Could you check a few things on this model? Use its own coordinates, in mm. A direction names the side the tool comes from. Give positions to 0.01 mm unless a question says otherwise; leave off trailing zeros. Write each loop counter-clockwise with the first axis right and the second up, starting at its lowest first coordinate (ties: lowest second). Pieces come first, ordered by that corner, then holes. Notation, with made-up numbers: (52.5, 47.5) - (77.5, 47.5) arc R17 cw to (77.5, 57.5) - close; hole circle Ø10 at (-30, -12.75). An arc over 180 degrees is marked (long way). Use one line per item in the form item = value.
```python
from build123d import *

# Parameters (mm, degrees)
BOSS_EXTRUDE1_DEPTH = 12.6
CUT_EXTRUDE1_DEPTH  = 7
CUT_EXTRUDE2_DEPTH  = 3
SKETCH5_R           = 1
BOSS_EXTRUDE2_DEPTH = 5.9
SKETCH6_R           = 1.25
BOSS_EXTRUDE3_DEPTH = 6.2
SKETCH7_R           = 0.85
CUT_EXTRUDE3_DEPTH  = 4.5
SKETCH8_W           = 3.3
SKETCH8_H           = 2.25
CUT_EXTRUDE4_DEPTH  = 18.024687956
CUT_EXTRUDE5_DEPTH  = 15.941218156
FILLET1_R           = 0.5
FILLET2_R           = 0.25
FILLET3_R           = 0.15
FILLET4_R           = 0.25


with BuildPart() as part:
    # Sketch1 → Boss-Extrude1 (new body)
    with BuildSketch(Plane(origin=(0, 0, 0), x_dir=(0, 0, -1), z_dir=(1, 0, 0))):
        Polygon((0, 0), (8.618070798, 0), (10.2, 1.6), (10.2, 3.6), (8.618070798, 5.2), (0, 5.2), align=None)
    extrude(amount=BOSS_EXTRUDE1_DEPTH)

    # Sketch2 → Cut-Extrude1 (cut)
    with BuildSketch(Plane(origin=(12.6, 0, 0), x_dir=(0, 0, -1), z_dir=(1, 0, 0))):
        Polygon((9.6, 3.353465579), (8.367544249, 4.6), (0.6, 4.6), (0.6, 0.6), (8.367544249, 0.6), (9.6, 1.846534421), align=None)
    extrude(amount=-CUT_EXTRUDE1_DEPTH, mode=Mode.SUBTRACT)

    # Sketch3 → Cut-Extrude2 (cut)
    with BuildSketch(Plane(origin=(0, 0, 0), x_dir=(0, 0, -1), z_dir=(1, 0, 0))):
        Polygon((9.6, 3.353465579), (8.367544249, 4.6), (0.6, 4.6), (0.6, 0.6), (8.367544249, 0.6), (9.6, 1.846534421), align=None)
    extrude(amount=CUT_EXTRUDE2_DEPTH, mode=Mode.SUBTRACT)

    # Sketch5 → Boss-Extrude2 (add)
    with BuildSketch(Plane(origin=(5.6, 0, 0), x_dir=(0, 0, -1), z_dir=(1, 0, 0))):
        with Locations((2.6, 2.6)):
            Circle(SKETCH5_R)
        with Locations((7.6, 2.6)):
            Circle(SKETCH5_R)
    extrude(amount=BOSS_EXTRUDE2_DEPTH)

    # Sketch6 → Boss-Extrude3 (add)
    with BuildSketch(Plane.ZY.offset(-3)):
        with Locations(Location((-7.6, 2.6, 0), (0, 0, 180))):
            Circle(SKETCH6_R)
        with Locations(Location((-2.6, 2.6, 0), (0, 0, 180))):
            Circle(SKETCH6_R)
    extrude(amount=BOSS_EXTRUDE3_DEPTH)

    # Sketch7 → Cut-Extrude3 (cut)
    with BuildSketch(Plane.ZY.offset(3.2)):
        with Locations((-7.6, 2.6)):
            Circle(SKETCH7_R)
        with Locations((-2.6, 2.6)):
            Circle(SKETCH7_R)
    extrude(amount=-CUT_EXTRUDE3_DEPTH, mode=Mode.SUBTRACT)

    # Sketch8 → Cut-Extrude4 (cut, through all)
    with BuildSketch(Plane(origin=(0, 5.2, 0), x_dir=(1, 0, 0), z_dir=(0, 1, 0))):
        with Locations((-2.55, 8.725)):
            Rectangle(SKETCH8_W, SKETCH8_H)
        with Locations((-2.55, 1.475)):
            Rectangle(SKETCH8_W, SKETCH8_H)
    extrude(amount=-CUT_EXTRUDE4_DEPTH, mode=Mode.SUBTRACT)

    # Sketch9 → Cut-Extrude5 (cut, through all)
    with BuildSketch(Plane.ZY.offset(-3)):
        with BuildLine():
            Line((-6.811013308, 4.6), (-3.388986692, 4.6))
            ThreePointArc((-3.388986692, 4.6), (-4.75, 2.6), (-3.388986692, 0.6))
            Line((-3.388986692, 0.6), (-6.811013308, 0.6))
            ThreePointArc((-6.811013308, 0.6), (-5.45, 2.6), (-6.811013308, 4.6))
        make_face()
    extrude(amount=-CUT_EXTRUDE5_DEPTH, mode=Mode.SUBTRACT)

    # Fillet1
    fillet1_edges = [part.edges().sort_by_distance(p)[0] for p in [
        (6.3, 5.2, 0),
        (6.3, 5.2, -8.618070798),
        (6.3, 3.6, -10.2),
        (6.3, 1.6, -10.2),
        (6.3, 0, -8.618070798),
        (6.3, 0, 0),
    ]]
    fillet(fillet1_edges, radius=FILLET1_R)

    # Fillet2
    fillet2_edges = [part.edges().sort_by_distance(p)[0] for p in [
        (9.1, 3.353465579, -9.6),
        (9.1, 1.846534421, -9.6),
        (9.1, 0.6, -8.367544249),
        (9.1, 0.6, -0.6),
        (9.1, 4.6, -0.6),
        (9.1, 4.6, -8.367544249),
        (1.5, 1.846534421, -9.6),
        (1.5, 3.353465579, -9.6),
        (1.5, 4.6, -8.367544249),
        (1.5, 4.6, -0.6),
        (1.5, 0.6, -0.6),
        (1.5, 0.6, -8.367544249),
    ]]
    fillet(fillet2_edges, radius=FILLET2_R)

    # Fillet3
    fillet3_edges = [part.edges().sort_by_distance(p)[0] for p in [
        (4.3, 0.6, -6.811013308),
        (4.3, 4.6, -6.811013308),
        (4.3, 4.6, -3.388986692),
        (4.3, 0.6, -3.388986692),
    ]]
    fillet(fillet3_edges, radius=FILLET3_R)

    # Fillet4
    fillet4_edges = [part.edges().sort_by_distance(p)[0] for p in [
        (11.5, 2.6, -1.6),
        (11.5, 2.6, -6.6),
    ]]
    fillet(fillet4_edges, radius=FILLET4_R)


solid = part.part
```
1. For pin 1 (1.5 mm diameter, centred on y = 2.6, z = -7.6, fed in from -X); pin 2 (1.2 mm diameter, centred on y = 3, z = -1.5, fed in from +X); pin 3 (0.6 mm diameter, centred on y = 3, z = -8.5, fed in from -X), each with a flat end and sliding along its axis, tell me the tip position at first contact or that it passes through.
Response values:
pin_1 = 1.3
pin_2 = 11.5
pin_3 = -0.9
2. If I drill on line 1 (Z direction, x = -0.2, y = 2.6); line 2 (Z direction, x = 0.2, y = 2.6); line 3 (Y direction, x = 10.75, z = -6.5), over which ranges is the centre line in solid material (lowest first)? Write a range as from..to.
Response values:
line_1 = -8.85..-8.45, -6.75..-6.35, -3.85..-3.45, -1.75..-1.35
line_2 = -10.2..-9.6, -8.85..-8.45, -6.75..-6.35, -3.85..-3.45, -1.75..-1.35, -0.6..0
line_3 = 0..0.6, 4.6..5.2
3. Imagine slicing it at C-C, the plane x = 5. List the corners of the cut face in (y, z) for me, and give its area (3 significant figures).
Response values:
outline = (0, -8.41) arc R0.5 ccw to (0.15, -8.76) - (1.45, -10.06) arc R0.5 ccw to (1.81, -10.2) - (3.39, -10.2) arc R0.5 ccw to (3.75, -10.06) - (5.05, -8.76) arc R0.5 ccw to (5.2, -8.41) - (5.2, -0.5) arc R0.5 ccw to (4.7, 0) - (0.5, 0) arc R0.5 ccw to (0, -0.5) - close; hole (0.6, -6.23) arc R0.15 ccw to (0.87, -6.32) arc R2.15 cw to (4.33, -6.32) arc R0.15 ccw to (4.6, -6.23) - (4.6, -3.97) arc R0.15 ccw to (4.33, -3.88) arc R2.15 cw to (0.87, -3.88) arc R0.15 ccw to (0.6, -3.97) - close
area = 44.8 mm²
4. Imagine slicing it at A-A, the plane x = 7.25. List the corners of the cut face in (y, z) for me, and give its area (3 significant figures).
Response values:
outline = (0, -8.41) arc R0.5 ccw to (0.15, -8.76) - (1.45, -10.06) arc R0.5 ccw to (1.81, -10.2) - (3.39, -10.2) arc R0.5 ccw to (3.75, -10.06) - (5.05, -8.76) arc R0.5 ccw to (5.2, -8.41) - (5.2, -0.5) arc R0.5 ccw to (4.7, 0) - (0.5, 0) arc R0.5 ccw to (0, -0.5) - close; circle Ø2 at (2.6, -7.6); circle Ø2 at (2.6, -2.6); hole (0.6, -8.26) arc R0.25 ccw to (0.67, -8.44) - (1.77, -9.53) arc R0.25 ccw to (1.95, -9.6) - (3.25, -9.6) arc R0.25 ccw to (3.43, -9.53) - (4.53, -8.44) arc R0.25 ccw to (4.6, -8.26) - (4.6, -0.85) arc R0.25 ccw to (4.35, -0.6) - (0.85, -0.6) arc R0.25 ccw to (0.6, -0.85) - close
area = 22.2 mm²
5. Which directions (+Z, -Z, +X, -X, +Y, -Y) give clear straight access to the entire face, cutting with the end or side of a thin tool? Please do faces 1 (the face through (11.5, 3, -8)), 2 (the face through (-0.48, 2.64, -3.45)), 3 (the face through (4.28, 2.63, -4.75)).
Response values:
face_1 = +X
face_2 = -X
face_3 = +X, -X
6. If we mould it in two halves opening along Z, with no side actions, what happens to faces 4 (the face through (9, 3, -0.6)), 5 (the face through (-0.9, 2.62, -1.55)), 6 (the face through (1, 3, -0.6)), 7 (the face through (6.21, 0.79, -9.4))? For each: pulls with the +Z half, pulls with the -Z half, needs draft (parallel to the pull), parting line crosses it, or undercut.
Response values:
face_4 = undercut
face_5 = needs draft
face_6 = undercut
face_7 = pulls with the -Z half
7. Imagine slicing it at B-B, the plane z = -5. List the corners of the cut face in (x, y) for me.
Response values:
outline = (0, 0) - (12.6, 0) - (12.6, 0.6) - (0, 0.6) - close; (0, 4.6) - (12.6, 4.6) - (12.6, 5.2) - (0, 5.2) - close
